Design review of the part built by this model. Coordinates are the model's own, in mm. Give positions to 0.01 mm unless a question says otherwise; leave off trailing zeros. Write each loop counter-clockwise with the first axis right and the second up, starting at its lowest first coordinate (ties: lowest second). Pieces come first, ordered by that corner, then holes. Notation, with made-up numbers: (-6.75, -29.75) - (4.25, -29.75) arc R18 cw to (4.25, -23.75) - close; hole circle Ø10 at (29, 49.25). An arc over 180 degrees is marked (long way). Use a Markdown table: item, result. Add a question column.
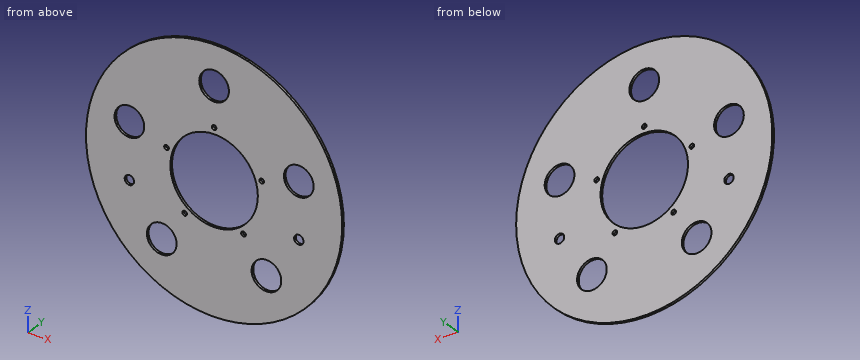
```python
from build123d import *

# Parameters (mm, degrees)
F0_R     = 82
F0_R_2   = 32
F0_R_3   = 28
F1_DEPTH = 1.5
F2_D     = 19
F3_D     = 6
F4_D     = 3


with BuildPart() as f1:
    # F0 (on Front) → F1 (new body)
    with BuildSketch(Plane.XZ):
        Circle(F0_R)
        Circle(F0_R_2, mode=Mode.SUBTRACT)
        Circle(F0_R_2)
        Circle(F0_R_3, mode=Mode.SUBTRACT)
    extrude(amount=-F1_DEPTH)

    # F2 (through all)
    with Locations(Plane.XZ):
        with Locations((0, 57), (54.2102264595, 17.6139531965), (33.5032664595, -46.1143268035), (-33.5032664595, -46.1143268035), (-54.2102264595, 17.6139531965)):
            Hole(F2_D / 2)

    # F3 (through all)
    with Locations(Plane.XZ):
        with Locations((-54.2102163981, -17.6139841623), (54.2102163981, -17.6139841623)):
            Hole(F3_D / 2)

    # F4 (through all)
    with Locations(Plane.XZ):
        with Locations((18.8088513457, -25.8887448722), (30.4338113457, 9.8885351278), (-18.8088513457, -25.8887448722), (-30.4338113457, 9.8885351278), (0, 32)):
            Hole(F4_D / 2)


solid = f1.part
```
(1) For line 1 along Z through (x, y) = (0, 0.8); line 2 along Z through (x, y) = (5.5, 0.25); line 3 along Z through (x, y) = (40, 0.4), list the stretches that pass through material, from the lowest coordinate up.
(2) Insertion check: pin 1 (1 mm diameter, centred on x = -40, z = -52, fed in from -Y). The pin has a flat end and moves straight along its axis. Give the tip position at first contact, or say it passes through.
(3) Add section B-B (y = 1.15). Count the separate pieces of the cut face and the enclosed holes in it, and give its area (3 significant figures).
(4) Add section C-C (z = 69). State the section outline as (x, y) points, and give its area (3 significant figures).
(5) Add section A-A (z = 0). State the section outline as (x, y) points, and give its area (3 significant figures).
Answers follow:
| question | item | result |
|---|---|---|
| 1 | line 1 | -82 to -28, 28 to 30.5, 33.5 to 47.5, 66.5 to 82 |
| 1 | line 2 | -81.82 to -27.45, 27.45 to 49.25, 64.75 to 81.82 |
| 1 | line 3 | -71.58 to -53.05, -39.18 to 71.58 |
| 2 | pin 1 | through |
| 3 | separate pieces | 1 |
| 3 | enclosed holes | 13 |
| 3 | area | 17,200 mm^2 |
| 4 | outline | (-44.31, 0) - (44.31, 0) - (44.31, 1.5) - (-44.31, 1.5) - close |
| 4 | area | 133 mm^2 |
| 5 | outline | (-82, 0) - (-28, 0) - (-28, 1.5) - (-82, 1.5) - close; (28, 0) - (82, 0) - (82, 1.5) - (28, 1.5) - close |
| 5 | area | 162 mm^2 |
